Geometry: final body of the model. Coordinates: model frame, mm. A direction names the side the tool comes from. Give positions to 0.01 mm unless a question says otherwise; leave off trailing zeros. Order: outer loops, then holes, each group sorted by start corner. A loop starts at its lowest first (then second) coordinate and runs counter-clockwise, first axis right, second up. Notation, with made-up numbers: (33.25, 58.5) - (77.25, 58.5) arc R33 ccw to (77.25, 95.5) - close; hole circle Ø8 at (0, 49.5). An arc over 180 degrees is marked (long way). Put each result on its own line as item: value. Start each with the question number.
1. First-contact query: P1, Ø1, axis at y = 2, z = -1, coming from the +X side. Flat tip, straight axial feed; report the tip coordinate or a pass-through.
2. Section B-B on y = 1.35. Return the cut outline in (x, z), plus the area to 3 significant figures.
3. Section A-A on z = 0. Return the cut outline in (x, y), plus the area to 3 significant figures.
4. Set-up query: faces 1 (the flat face through (-25, 1, -1.6)), 2 (the flat face through (-15, 1, -3.5)). Return all of +Z, -Z, +X, -X, +Y, -Y with unobstructed straight access to the full face (end or side cutting, diameter ignored); none if empty.
5. Ray query, line 1 along X through (y, z) = (1.45, 0); line 2 along Z through (x, y) = (0, 0.6); line 3 along X through (y, z) = (1.7, -0.5). Return the intervals inside material, ascending. Write a range as from..to.
6. Mould query, pull axis Z, two halves, no side actions, for faces 3 (the cylindrical face through (-1.27, 0.99, 0.97)), 4 (the flat face through (-15, 3, 0)), 5 (the cylindrical face through (3.5, 1.5, -0.1)), 6 (the cylindrical face through (-31.6, 1.5, 0)). Classes: pulls with the +Z half, pulls with the -Z half, needs draft (parallel to the pull), parting line crosses it, or undercut.
from build123d import *

# Parameters (mm, degrees)
SKETCH_1_R      = 1.6
EXTRUDE_1_DEPTH = 3
CHAMFER_1_SIZE  = 1


with BuildPart() as part:
    # Эскиз1 → Бобышка-Вытянуть1 (new body)
    with BuildSketch(Plane(origin=(0, 0, 0), x_dir=(1, 0, 0), z_dir=(0, 1, 0))):
        with BuildLine():
            Line((-30, 3.5), (0, 3.5))
            ThreePointArc((0, 3.5), (3.5, 0), (0, -3.5))
            Line((0, -3.5), (-30, -3.5))
            ThreePointArc((-30, -3.5), (-33.5, 0), (-30, 3.5))
        make_face()
        Circle(SKETCH_1_R, mode=Mode.SUBTRACT)
        with BuildLine():
            Line((-30, 1.6), (-20, 1.6))
            ThreePointArc((-20, 1.6), (-18.4, 0), (-20, -1.6))
            Line((-20, -1.6), (-30, -1.6))
            ThreePointArc((-30, -1.6), (-31.6, 0), (-30, 1.6))
        make_face(mode=Mode.SUBTRACT)
    extrude(amount=EXTRUDE_1_DEPTH)

    # Фаска1
    chamfer_1_edges = [part.edges().sort_by_distance(p)[0] for p in [
        (-1.6, 3, 0),
    ]]
    chamfer(chamfer_1_edges, length=CHAMFER_1_SIZE)


solid = part.part
Resolved:
1. P1: x = 3.46
2. outline: (-30, -3.5) - (0, -3.5) arc R3.5 ccw to (0, 3.5) - (-30, 3.5) arc R3.5 ccw to start; hole (-30, -1.6) - (-20, -1.6) arc R1.6 ccw to (-20, 1.6) - (-30, 1.6) arc R1.6 ccw to start; hole circle Ø3.2 at (0, 0)
2. area: 200 mm^2
3. outline: (-33.5, 0) - (-31.6, 0) - (-31.6, 3) - (-33.5, 3) - close; (-18.4, 0) - (-1.6, 0) - (-1.6, 2) - (-2.6, 3) - (-18.4, 3) - close; (1.6, 0) - (3.5, 0) - (3.5, 3) - (2.6, 3) - (1.6, 2) - close
3. area: 60.8 mm^2
4. face 1: +Y, -Y
4. face 2: -Z, +X, -X, +Y, -Y
5. line 1: -33.5..-31.6, -18.4..-1.6, 1.6..3.5
5. line 2: -3.5..-1.6, 1.6..3.5
5. line 3: -33.46..-31.52, -18.48..-1.52, 1.52..3.46
6. face 3: undercut
6. face 4: needs draft
6. face 5: parting line crosses it
6. face 6: undercut
